from build123d import *

# Parameters (mm, degrees)
SKETCH1_W           = 400
SKETCH1_H           = 50
BOSS_EXTRUDE1_DEPTH = 65
SKETCH2_R           = 5
CUT_EXTRUDE1_DEPTH  = 66


with BuildPart() as part:
    # Sketch1 → Boss-Extrude1 (new body)
    with BuildSketch(Plane(origin=(0, 0, 0), x_dir=(0, 0, -1), z_dir=(1, 0, 0))):
        Rectangle(SKETCH1_W, SKETCH1_H)
    extrude(amount=BOSS_EXTRUDE1_DEPTH)

    # Sketch2 → Cut-Extrude1 (cut, through all)
    with BuildSketch(Plane(origin=(65, 0, 0), x_dir=(0, 0, -1), z_dir=(1, 0, 0))):
        with Locations((-180, 0)):
            Circle(SKETCH2_R)
        with Locations((-160, 0)):
            Circle(SKETCH2_R)
        with Locations((-140, 0)):
            Circle(SKETCH2_R)
        with Locations((-120, 0)):
            Circle(SKETCH2_R)
        with Locations((-100, 0)):
            Circle(SKETCH2_R)
        with Locations((-80, 0)):
            Circle(SKETCH2_R)
        with Locations((-60, 0)):
            Circle(SKETCH2_R)
        with Locations((-40, 0)):
            Circle(SKETCH2_R)
        with Locations((-20, 0)):
            Circle(SKETCH2_R)
        Circle(SKETCH2_R)
        with Locations((20, 0)):
            Circle(SKETCH2_R)
        with Locations((40, 0)):
            Circle(SKETCH2_R)
        with Locations((60, 0)):
            Circle(SKETCH2_R)
        with Locations((80, 0)):
            Circle(SKETCH2_R)
        with Locations((100, 0)):
            Circle(SKETCH2_R)
        with Locations((120, 0)):
            Circle(SKETCH2_R)
        with Locations((140, 0)):
            Circle(SKETCH2_R)
        with Locations((160, 0)):
            Circle(SKETCH2_R)
        with Locations((180, 0)):
            Circle(SKETCH2_R)
    extrude(amount=-CUT_EXTRUDE1_DEPTH, mode=Mode.SUBTRACT)


solid = part.part
CAD build for the part. Positions are in the model's coordinates, mm. Round coordinates to 2 decimals unless told otherwise and drop trailing zeros. Order: outer loops, then holes, each group sorted by start corner. A loop starts at its lowest first (then second) coordinate and runs counter-clockwise, first axis right, second up. Notation, with made-up numbers: (81.5, -3.75) -> (111.5, -3.75) arc R28 ccw to (111.5, 18.25) -> close; hole circle Ø5 at (6, 10). An arc over 180 degrees is marked (long way). Write each question's results on one line, items separated by ' | '.
1. Flat gauge pin, fed straight in: P1, Ø6, axis at y = 0, z = -80, coming from the +X side. Where does the tip first touch, or does it go through?
Findings below:
P1: passes through
2. Pull direction Y, two halves, no side cores. Call faces 1 (the face through (33, 0, -55)), 2 (the face through (32, -25, 3)), 3 (the face through (65, 6, 3)): pulls with the +Y half, pulls with the -Y half, needs draft (parallel to the pull), parting line crosses it, or undercut.
Findings below:
face 1: undercut | face 2: pulls with the -Y half | face 3: needs draft
3. Cut at A-A (x = 42.5). Count the separate pieces of the cut face and the enclosed holes in it, plus the area to 3 significant figures.
Findings below:
separate pieces: 1 | enclosed holes: 19 | area: 18,500 mm²
4. Wall check: line 1 along Y through (x, z) = (13, 20); line 2 along Y through (x, z) = (43, -63). Give the ranges that are in metal, low to high. Write a range as [from, to].
Findings below:
line 1: y = [-25, -5], [5, 25] | line 2: y = [-25, -4], [4, 25]
5. Cut at B-B (z = 60). Give the cut face in (x, y).
Findings below:
outline: (0, -25) -> (65, -25) -> (65, -5) -> (0, -5) -> close; (0, 5) -> (65, 5) -> (65, 25) -> (0, 25) -> close
